Autodesk Inventor part; units mm, degrees
ref_plane "YZ Plane" through (0, 0, 0) normal (1, 0, 0) x (0, 1, 0)
ref_plane "XZ Plane" through (0, 0, 0) normal (0, 1, 0) x (-1, 0, 0)
ref_plane "XY Plane" through (0, 0, 0) normal (0, 0, 1) x (1, 0, 0)
sketch "Sketch1" plane through (0, 0, 0) normal (0, 0, 1) x (1, 0, 0)
  line L0 (0, 0) -> (100, 0)
  line L1 (100, 0) -> (100, 94)
  line L2 (100, 94) -> (0, 94)
  line L3 (0, 94) -> (0, 0)
  dimension "d0" = 100
  dimension "d1" = 94
extrude "Extrusion1" add sketch "Sketch1" along normal blind 3
sketch "Sketch2" plane through (0, 0, 3) normal (0, 0, 1) x (1, 0, 0)
  line L0 (100, 94) -> (0, 94)
  line L1 (8.25, 94) -> (91.75, 94)
  line L2 (91.75, 94) -> (91.75, 0)
  line L3 (91.75, 0) -> (8.25, 0)
  line L4 (8.25, 0) -> (8.25, 94)
  line L5 (100, 0) -> (100, 94) construction
  line L6 (100, 94) -> (92, 94) construction
  line L7 (92, 94) -> (92, 0) construction
  line L8 (92, 0) -> (100, 0) construction
  line L9 (100, 0) -> (100, 94) construction
  line L10 (0, 94) -> (8, 94) construction
  line L11 (8, 94) -> (8, 0) construction
  line L12 (8, 0) -> (0, 0) construction
  line L13 (0, 0) -> (0, 94) construction
  line L14 (0, 0) -> (100, 0) construction
  dimension "d4" = 8
  dimension "d5" = 0.25
  dimension "d6" = 0.25
extrude "Extrusion2" add sketch "Sketch2" along normal blind 2
sketch "Sketch4" plane through (0, 0, 0) normal (0, -1, 0) x (1, 0, 0)
  line L0 (91.75, 5) -> (8.25, 5)
  line L1 (8.25, 5) -> (91.75, 5)
  line L2 (91.75, 5) -> (91.75, 8)
  line L3 (91.75, 8) -> (8.25, 8)
  line L4 (8.25, 8) -> (8.25, 5)
  line L5 (91.75, 3) -> (91.75, 5)
  line L6 (0, 0) -> (100, 0)
  dimension "d10" = 8
extrude "Extrusion3" add sketch "Sketch4" against normal blind 3
sketch "Sketch6" plane through (0, 0, 0) normal (0, -1, 0) x (1, 0, 0)
  line L0 (0, 0) -> (100, 0)
  line L1 (91.75, 8) -> (8.25, 8)
  line L2 (100, 0) -> (100, 3)
  point P0 (25, 4)
  point P1 (75, 4)
  dimension "d20" = 8
  dimension "d21" = 4
  dimension "d22" = 100
  dimension "d23" = 25
  dimension "d24" = 50
hole "Hole1" at (25, 0, 4) at (75, 0, 4) direction (0, 1, 0) diameter 2.459 depth 3.5 tip angle 118
sketch "Sketch7" plane through (0, 0, 0) normal (0, 0, -1) x (-1, 0, 0)
  line L0 (-91.75, 94) -> (-91.75, 0)
  line L1 (-8.25, 0) -> (-8.25, 94)
  line L2 (-100, 0) -> (-100, 94)
  line L3 (0, 94) -> (0, 0)
  line L4 (-100, 94) -> (0, 94)
  point P0 (-96, 70.5)
  point P1 (-4, 70.5)
  point P2 (-96, 23.5)
  point P3 (-4, 23.5)
  dimension "d32" = 8.25
  dimension "d33" = 4
  dimension "d34" = 4
  dimension "d35" = 94
  dimension "d36" = 23.5
  dimension "d39" = 47
hole "Hole2" at (96, 70.5, 0) at (4, 70.5, 0) at (96, 23.5, 0) at (4, 23.5, 0) direction (0, 0, 1) diameter 2.2 depth 3.5 tip angle 118 countersink diameter 4.4 countersink angle 90
chamfer "Chamfer2" distance 0.5 angle 45 3 edges at (8.25, 48.5, 5) (50, 3, 8) (91.75, 48.5, 5)
chamfer "Chamfer3" distance 1 angle 45 1 edges at (50, 94, 5)
chamfer "Chamfer4" distance 1 angle 45 2 edges at (100, 47, 0) (0, 47, 0)
equation "\"d6\" = d5"
properties part number "FrontPanel" material "Aluminum 6061"
Input: part model. Units: mm. Frame: model coordinates. A direction names the side the tool comes from. Give positions to 0.01 mm unless a question says otherwise; leave off trailing zeros. Order: outer loops, then holes, each group sorted by start corner. A loop starts at its lowest first (then second) coordinate and runs counter-clockwise, first axis right, second up. Notation, with made-up numbers: M 13.25,28.25 L 58.25,28.25 A14 cw 58.25,41.25 Z; hole C 0.25,27 d1. An arc over 180 degrees is marked long. One line per question, with ' | ' between items. Start each with the question number.
1. Material intervals for probe 1 along X at (y, z) = (2, 4); probe 2 along Y at (x, z) = (96, 2.45); probe 3 along X at (y, z) = (23.5, 2.6), sorted ascending. Write a range as [from, to].
2. Section query C-C (y = 53). Return the cut outline in (x, z).
3. Section query B-B (y = 70.5). Return the cut outline in (x, z).
4. Section query A-A (x = 4). Return the cut outline in (y, z), and give its area (3 significant figures).
5. Access query for faces 1 (the face through (74.631, 1.774, 2.827)), 2 (the face through (49, 49, 5)), 3 (the face through (8.25, 43, 4)), 4 (the face through (91.75, 43, 4)). Directions: +Z, -Z, +X, -X, +Y, -Y. A direction counts if a zero-diameter tool reaches every point of the face in a straight line with its end or side. Return the directions, or none.
6. First-contact query: pin 1 Ø12 at (x, y) = (80, 74) entering from +Z; pin 2 Ø1.5 at (y, z) = (24, 4) entering from -X; pin 3 Ø3 at (x, y) = (96, 70.5) entering from +Z. Flat tips, straight axial feed; report the tip coordinate or a pass-through.
7. Section query D-D (x = 28.5). Return the cut outline in (y, z), and give its area (3 significant figures).
8. Pull-direction query (Y, two-part tool) for faces 5 (the face through (25.471, 1.774, 2.864)), 6 (the face through (49, 0, 4)), 7 (the face through (4, 22.4, 2.1)); classes: released by +Y, released by -Y, zero draft, split by the parting line, or undercut.
Here are the results:
1) probe 1: [8.25, 23.77], [26.23, 73.77], [76.23, 91.75] | probe 2: [0, 22.4], [24.6, 69.4], [71.6, 94] | probe 3: [0, 2.9], [5.1, 94.9], [97.1, 100]
2) outline: M 0,1 L 1,0 L 99,0 L 100,1 L 100,3 L 91.75,3 L 91.75,4.5 L 91.25,5 L 8.75,5 L 8.25,4.5 L 8.25,3 L 0,3 Z
3) outline: M 0,1 L 1,0 L 1.8,0 L 2.9,1.1 L 2.9,3 L 0,3 Z; M 5.1,1.1 L 6.2,0 L 93.8,0 L 94.9,1.1 L 94.9,3 L 91.75,3 L 91.75,4.5 L 91.25,5 L 8.75,5 L 8.25,4.5 L 8.25,3 L 5.1,3 Z; M 97.1,1.1 L 98.2,0 L 99,0 L 100,1 L 100,3 L 97.1,3 Z
4) outline: M 0,0 L 21.3,0 L 22.4,1.1 L 22.4,3 L 0,3 Z; M 24.6,1.1 L 25.7,0 L 68.3,0 L 69.4,1.1 L 69.4,3 L 24.6,3 Z; M 71.6,1.1 L 72.7,0 L 94,0 L 94,3 L 71.6,3 Z | area: 266 mm²
5) face 1: -Y | face 2: +Z, +X, -X, +Y | face 3: +Z, -X, +Y, -Y | face 4: +Z, +X, +Y, -Y
6) pin 1: z = 5 | pin 2: x = 8.25 | pin 3: z = 3
7) outline: M 0,0 L 94,0 L 94,4 L 93,5 L 3,5 L 3,7.5 L 2.5,8 L 0,8 Z | area: 478 mm²
8) face 5: zero draft | face 6: released by -Y | face 7: undercut
